Autodesk Inventor part; units mm, degrees
ref_plane "YZ Plane" through (0, 0, 0) normal (1, 0, 0) x (0, 1, 0)
ref_plane "XZ Plane" through (0, 0, 0) normal (0, 1, 0) x (-1, 0, 0)
ref_plane "XY Plane" through (0, 0, 0) normal (0, 0, 1) x (1, 0, 0)
sketch "Sketch1" plane through (0, 0, 0) normal (0, 0, 1) x (1, 0, 0)
  line L0 (14.98, 33.7) -> (197.7852, 33.7)
  line L1 (197.7852, 8.3) -> (14.98, 8.3)
  line L2 (14.98, 8.3) -> (14.98, 33.7)
  arc A0 (30.1177, 21.5547) -> (28.8951, 18.8151) centre (27.68, 21) ccw
  line L3 (30.1177, 21.5547) -> (28.8951, 18.8151)
  line L4 (-3.175, 42) -> (-122.9515, 42)
  line L5 (137.6968, 28.62) -> (137.6968, 13.38)
  line L6 (137.6968, 13.38) -> (122.4568, 28.62)
  line L7 (122.4568, 28.62) -> (137.6968, 28.62)
  line L8 (130.5126, 13.38) -> (115.2726, 28.62)
  line L9 (115.2726, 28.62) -> (115.2726, 13.38)
  line L10 (115.2726, 13.38) -> (130.5126, 13.38)
  line L11 (112.7326, 10.7487) -> (112.7326, 41.4812) construction
  line L12 (87.7684, 28.62) -> (87.7684, 13.38)
  line L13 (87.7684, 13.38) -> (103.0084, 28.62)
  line L14 (103.0084, 28.62) -> (87.7684, 28.62)
  line L15 (94.9526, 13.38) -> (110.1926, 28.62)
  line L16 (110.1926, 28.62) -> (110.1926, 13.38)
  line L17 (110.1926, 13.38) -> (94.9526, 13.38)
  line L18 (85.2284, 8.9371) -> (85.2284, 32.7241) construction
  line L19 (32.76, 28.62) -> (32.76, 13.38)
  line L20 (32.76, 13.38) -> (48, 28.62)
  line L21 (48, 28.62) -> (32.76, 28.62)
  line L22 (39.9442, 13.38) -> (55.1842, 28.62)
  line L23 (55.1842, 28.62) -> (55.1842, 13.38)
  line L24 (55.1842, 13.38) -> (39.9442, 13.38)
  line L25 (82.6884, 28.62) -> (82.6884, 13.38)
  line L26 (82.6884, 13.38) -> (67.4484, 28.62)
  line L27 (67.4484, 28.62) -> (82.6884, 28.62)
  line L28 (75.5042, 13.38) -> (60.2642, 28.62)
  line L29 (60.2642, 13.38) -> (75.5042, 13.38)
  line L30 (60.2642, 28.62) -> (60.2642, 13.38)
  line L31 (140.2368, 33.7) -> (140.2368, 8.3) construction
  line L32 (142.7768, 28.62) -> (142.7768, 13.38)
  line L33 (142.7768, 13.38) -> (158.0168, 28.62)
  line L34 (158.0168, 28.62) -> (142.7768, 28.62)
  line L35 (149.961, 13.38) -> (165.201, 28.62)
  line L36 (165.201, 28.62) -> (165.201, 13.38)
  line L37 (165.201, 13.38) -> (149.961, 13.38)
  line L38 (192.7052, 28.62) -> (192.7052, 13.38)
  line L39 (192.7052, 13.38) -> (177.4652, 28.62)
  line L40 (177.4652, 28.62) -> (192.7052, 28.62)
  line L41 (185.521, 13.38) -> (170.281, 28.62)
  line L42 (170.281, 13.38) -> (185.521, 13.38)
  line L43 (170.281, 28.62) -> (170.281, 13.38)
  line L44 (197.7852, 33.7) -> (197.7852, 8.3)
  point P0 (0, 0)
  dimension "d0" = 12.7
  dimension "d1" = 12.7
  dimension "d2" = 12.7
  dimension "d7" = 45
  dimension "d9" = 5.08
  dimension "d10" = 5.08
  dimension "d11" = 5.08
  dimension "d12" = 0
  dimension "d14" = 2.54
  dimension "d15" = 2.54
  dimension "d16" = 5.08
  dimension "d23" = 2.54
  dimension "d24" = 5.08
extrude "Extrusion3" add sketch "Sketch1" along normal blind 6.35
fillet "Fillet5" radius 3.175 12 edges at (165.201, 13.38, 3.175) (170.281, 13.38, 3.175) (192.7052, 28.62, 3.175) (142.7768, 28.62, 3.175) (137.6968, 28.62, 3.175) (115.2726, 13.38, 3.175) (110.1926, 13.38, 3.175) (87.7684, 28.62, 3.175) (82.6884, 28.62, 3.175) (60.2642, 13.38, 3.175) (55.1842, 13.38, 3.175) (32.76, 28.62, 3.175)
fillet "Fillet6" radius 3.175 12 edges at (106.3826, 33.7, 6.35) (106.3826, 33.7, 0) (197.7852, 33.7, 3.175) (197.7852, 21, 6.35) (197.7852, 21, 0) (197.7852, 8.3, 3.175) (106.3826, 8.3, 6.35) (106.3826, 8.3, 0) (14.98, 21, 0) (14.98, 33.7, 3.175) (14.98, 21, 6.35) (14.98, 8.3, 3.175)
equation "\"d1\" = d0"
equation "\"d24\" = d9"
properties part number "endarm"
Build history of the part. All positions in model axes, mm. A direction names the side the tool comes from. Coordinates: 2 decimals unless noted, no trailing zeros.
1. 3-axis set-ups, long thin cutter, end or side, ignore diameter. For faces 4 (the cylindrical face through (107.62, 32.75, 0.91)), 5 (the flat face through (95.28, 20.89, 3.13)): which of +Z, -Z, +X, -X, +Y, -Y reach the whole face in a straight line?
Answer block:
face 4: -Z, +X, -X, +Y
face 5: +Z, -Z
2. Pull direction X, two halves, no side cores. Call faces 1 (the cylindrical face through (105.15, 9.21, 5.4)), 2 (the cylindrical face through (196.831, 20.867, 0.905)), 3 (the cylindrical face through (33.7, 27.7, 3.2)): released by +X, released by -X, zero draft, split by the parting line, or undercut.
Answer block:
face 1: zero draft
face 2: released by +X
face 3: undercut
3. Band-saw the part on A-A, the plane x = 154. Give the number of separate pieces and of enclosed holes in the cut face, and give its area (3 significant figures).
Answer block:
separate pieces: 3
enclosed holes: 0
area: 101 mm2
4. Drop flat-ended pins along their axis: pin 1 (1.9 mm diameter, centred on x = 99.5, z = 2, fed in from +Y); pin 2 (1.9 mm diameter, centred on y = 21.5, z = 4.5, fed in from -X). Give the stop position or say it passes through.
Answer block:
pin 1: stops at y = 33.69
pin 2: stops at x = 15
5. Drill centre lines: probe 1 along Y at (x, z) = (127.5, 2.5); probe 2 along Y at (x, z) = (43.5, 3.75); probe 3 along Y at (x, z) = (91, 2). Where is each one in solid material? Low to high.
Answer block:
probe 1: y = 8.37 to 13.38, 16.39 to 23.58, 28.62 to 33.63
probe 2: y = 8.35 to 13.38, 16.94 to 24.12, 28.62 to 33.65
probe 3: y = 8.53 to 16.61, 28.62 to 33.47
